Model file for the job. Use its own axes, mm. A direction names the side the tool comes from. Give positions to 0.01 mm unless a question says otherwise; leave off trailing zeros. Order: outer loops, then holes, each group sorted by start corner. A loop starts at its lowest first (then second) coordinate and runs counter-clockwise, first axis right, second up. Notation, with made-up numbers: (66.25, 50.25) -> (88.25, 50.25) arc R17 cw to (88.25, 63.25) -> close; hole circle Ø5 at (62, 83.5). An arc over 180 degrees is marked (long way). Use CSV: the item, a comma, the result in double quotes. Start each with the question number.
1. Cut at D-D on y = 15.6. List the corners of the cut face in (x, z).
2. 3-axis set-ups, long thin cutter, end or side, ignore diameter. For faces 1 (the flat face through (2, 16, 0)), 2 (the flat face through (9, 5.7, 7)), 3 (the flat face through (3, 9, 7)), 4 (the cylindrical face through (3.65, 17.53, -1.48)): which of +Z, -Z, +X, -X, +Y, -Y reach the whole face in a straight line?
3. Cut at B-B on y = 1.25. List the corners of the cut face in (x, z).
4. Pull direction X, two halves, no side cores. Call faces 5 (the flat face through (14, 9, 7)), 6 (the flat face through (8, 0, 1)), 7 (the cylindrical face through (1.68, 14.31, 0.79)), 8 (the cylindrical face through (14.98, 14.31, 0.79)): released by +X, released by -X, zero draft, split by the parting line, or undercut.
5. Wall check: line 1 (X direction, y = 15.6, z = 0.5); line 2 (Y direction, x = 1.85, z = 0.45); line 3 (X direction, y = 15, z = 0.25). Give the ranges that are in metal, low to high. Write a range as from..to.
6. Drop flat-ended pins along their axis: pin 1 (8 mm diameter, centred on x = 6.5, z = 6, fed in from -Y); pin 2 (6 mm diameter, centred on y = 12, z = 8.5, fed in from +X); pin 3 (2.5 mm diameter, centred on x = 1.85, y = 15.6, fed in from +Z). Give the stop position or say it passes through.
7. Cut at C-C on z = 9.75. List the corners of the cut face in (x, y), then the cut area to 3 significant figures.
Autodesk Inventor part; units mm, degrees
ref_plane "YZ Plane" through (0, 0, 0) normal (1, 0, 0) x (0, 1, 0)
ref_plane "XZ Plane" through (0, 0, 0) normal (0, 1, 0) x (-1, 0, 0)
ref_plane "XY Plane" through (0, 0, 0) normal (0, 0, 1) x (1, 0, 0)
sketch "Sketch1" plane through (0, 0, 0) normal (0, 0, 1) x (1, 0, 0)
  line L0 (0, 0) -> (17, 0)
  line L1 (17, 0) -> (17, 17.6)
  line L2 (17, 17.6) -> (0, 17.6)
  line L3 (0, 17.6) -> (0, 0)
  circle A0 centre (16.25, 16.85) radius 0.75
  circle A1 centre (0.75, 16.85) radius 0.75
  circle A2 centre (0.75, 0.75) radius 0.75
  circle A3 centre (16.25, 0.75) radius 0.75
  circle A4 centre (1.85, 15.6) radius 1.3
  circle A5 centre (15.15, 15.6) radius 1.3
  circle A6 centre (8.5, 2) radius 1.3
  point P0 (0, 16.85)
  point P1 (0, 0.75)
  point P2 (0.75, 0)
  point P3 (16.25, 0)
  point P4 (17, 0.75)
  point P5 (17, 16.85)
  point P6 (16.25, 17.6)
  point P7 (0.75, 17.6)
  dimension "d0" = 17
  dimension "d1" = 17.6
  dimension "d2" = 1.5
  dimension "d3" = 1.5
  dimension "d4" = 1.5
  dimension "d5" = 1.5
  dimension "d7" = 2.6
  dimension "d11" = 1.85
  dimension "d12" = 1.85
  dimension "d13" = 2
  dimension "d14" = 2.6
  dimension "d15" = 2
  dimension "d16" = 8.5
extrude "Extrusion1" add sketch "Sketch1" along normal blind 1.6 contours A2 L3 A1 A4 L2 A0 A5 L1 A3 L0 | A2 | A3 | A1 A4 | A0 A5 picked at (1.0458, 16.9665) picked at (15.9541, 16.9666)
sketch "Sketch2" plane through (0, 0, 1.6) normal (0, 0, 1) x (1, 0, 0)
  line L0 (3, 11.9) -> (14, 11.9)
  line L1 (14, 11.9) -> (14, 5.7)
  line L2 (14, 5.7) -> (3, 5.7)
  line L3 (3, 5.7) -> (3, 11.9)
  line L4 (3, 11.9) -> (14, 5.7) construction
  line L5 (14, 11.9) -> (3, 5.7) construction
  line L6 (0, 16.85) -> (0, 0.75)
  line L7 (16.25, 17.6) -> (0.75, 17.6)
  point P0 (0, 0)
  point P1 (8.5, 8.8)
  point P2 (0, 8.8)
  point P3 (8.5, 17.6)
  point P4 (0, 8.8)
  point P5 (8.5, 5.7)
  dimension "d19" = 11
  dimension "d20" = 6.2
extrude "Extrusion2" add sketch "Sketch2" along normal blind 10
sketch "Sketch3" plane through (0, 0, 0) normal (0, 0, -1) x (-1, 0, 0)
  circle A0 centre (-14, 14.6) radius 3
  circle A1 centre (-3, 14.6) radius 3
  circle A2 centre (-8.5, 3) radius 3
  circle A3 centre (-8.5, 2) radius 1.3
  line L0 (-0.75, 0) -> (-16.25, 0)
  line L1 (-16.25, 17.6) -> (-0.75, 17.6)
  line L2 (-17, 0.75) -> (-17, 16.85)
  line L3 (0, 16.85) -> (0, 0.75)
  point P0 (0, 0)
  dimension "d23" = 6
  dimension "d24" = 6
  dimension "d25" = 6
extrude "Extrusion3" add sketch "Sketch3" along normal blind 3 contours A0 | A1 | A2 | A3
equation "\"d12\" = d11"
properties part number "clicky pcb top"
Verdict:
1,outline,"(0, 0) -> (0.17, 0) -> (0.17, -3) -> (5.83, -3) -> (5.83, 0) -> (11.17, 0) -> (11.17, -3) -> (16.83, -3) -> (16.83, 0) -> (17, 0) -> (17, 1.6) -> (16.45, 1.6) -> (16.45, 0) -> (13.85, 0) -> (13.85, 1.6) -> (3.15, 1.6) -> (3.15, 0) -> (0.55, 0) -> (0.55, 1.6) -> (0, 1.6) -> close"
2,face 1,"+Z"
2,face 2,"+Z, +X, -X, -Y"
2,face 3,"+Z, -X, +Y, -Y"
2,face 4,"-Z"
3,outline,"(0, 0) -> (6.06, 0) -> (6.06, -3) -> (10.94, -3) -> (10.94, 0) -> (17, 0) -> (17, 1.6) -> (9.56, 1.6) -> (9.56, 0) -> (7.44, 0) -> (7.44, 1.6) -> (0, 1.6) -> close"
4,face 5,"released by +X"
4,face 6,"zero draft"
4,face 7,"undercut"
4,face 8,"undercut"
5,line 1,"0..0.55, 3.15..13.85, 16.45..17"
5,line 2,"0..14.3, 16.9..17.6"
5,line 3,"0..0.7, 3..14, 16.3..17"
6,pin 1,"y = 5.7"
6,pin 2,"x = 14"
6,pin 3,"z = 0"
7,outline,"(3, 5.7) -> (14, 5.7) -> (14, 11.9) -> (3, 11.9) -> close"
7,area,"68.2 mm^2"
